from build123d import *

# Parameters (mm, degrees)
CYLINDER002_R     = 18.75
CYLINDER002_DEPTH = 1.4
CYLINDER001_R     = 18.6
CYLINDER001_DEPTH = 2.2
SKETCH_R          = 18.7
PAD_DEPTH         = 24
SKETCH001_R       = 16
PAD001_DEPTH      = 30
SKETCH002_R       = 1
PAD002_DEPTH      = 12
SKETCH003_R       = 13
PAD003_DEPTH      = 16
SKETCH004_R       = 17.5
PAD004_DEPTH      = 11
SKETCH008_R       = 22
SKETCH008_R_2     = 12
PAD008_DEPTH      = 2.5
SKETCH007_R       = 22
SKETCH007_R_2     = 12
PAD007_DEPTH      = 2.5
SKETCH006_R       = 22
SKETCH006_R_2     = 16
PAD006_DEPTH      = 2.5
SKETCH005_R       = 22
SKETCH005_R_2     = 16
PAD005_DEPTH      = 2.5
CYLINDER_R        = 20
CYLINDER_DEPTH    = 93


with BuildPart() as obj1:
    # Cylinder002 → Cylinder002 (new body)
    with BuildSketch(Plane.XY.offset(90)):
        Circle(CYLINDER002_R)
    extrude(amount=CYLINDER002_DEPTH)


with BuildPart() as nut_radial:
    # Cylinder001 → Cylinder001 (new body)
    with BuildSketch(Plane.XY.offset(84)):
        Circle(CYLINDER001_R)
    extrude(amount=CYLINDER001_DEPTH)


with BuildPart() as obj2:
    # Sketch → Pad (new body)
    with BuildSketch(Plane.XY):
        Circle(SKETCH_R)
    extrude(amount=PAD_DEPTH)

    # Sketch001 → Pad001 (new body)
    with BuildSketch(Plane.XY.offset(24)):
        Circle(SKETCH001_R)
    extrude(amount=PAD001_DEPTH)

    # Sketch002 → Pad002 (new body)
    with BuildSketch(Plane.XY.offset(54)):
        with Locations((-9.2, 0)):
            Circle(SKETCH002_R)
    extrude(amount=PAD002_DEPTH)

    # Sketch003 → Pad003 (new body)
    with BuildSketch(Plane.XY.offset(66)):
        Circle(SKETCH003_R)
    extrude(amount=PAD003_DEPTH)

    # Sketch004 → Pad004 (new body)
    with BuildSketch(Plane.XY.offset(82)):
        Circle(SKETCH004_R)
    extrude(amount=PAD004_DEPTH)


with BuildPart() as pad008:
    # Sketch008 → Pad008 (new body)
    with BuildSketch(Plane.XY.offset(56)):
        Circle(SKETCH008_R)
        Circle(SKETCH008_R_2, mode=Mode.SUBTRACT)
    extrude(amount=PAD008_DEPTH)


with BuildPart() as pad007:
    # Sketch007 → Pad007 (new body)
    with BuildSketch(Plane.XY.offset(61)):
        Circle(SKETCH007_R)
        Circle(SKETCH007_R_2, mode=Mode.SUBTRACT)
    extrude(amount=PAD007_DEPTH)


with BuildPart() as pad006:
    # Sketch006 → Pad006 (new body)
    with BuildSketch(Plane.XY.offset(71)):
        Circle(SKETCH006_R)
        Circle(SKETCH006_R_2, mode=Mode.SUBTRACT)
    extrude(amount=PAD006_DEPTH)


with BuildPart() as pad005:
    # Sketch005 → Pad005 (new body)
    with BuildSketch(Plane.XY.offset(66)):
        Circle(SKETCH005_R)
        Circle(SKETCH005_R_2, mode=Mode.SUBTRACT)
    extrude(amount=PAD005_DEPTH)


with BuildPart() as cut012:
    # Cylinder → Cylinder (new body)
    with BuildSketch(Plane.XY):
        Circle(CYLINDER_R)
    extrude(amount=CYLINDER_DEPTH)

    # Cut: cut Pad005
    add(pad005.part, mode=Mode.SUBTRACT)

    # Cut001: cut Pad006
    add(pad006.part, mode=Mode.SUBTRACT)

    # Cut002: cut Pad007
    add(pad007.part, mode=Mode.SUBTRACT)

    # Cut003: cut Pad008
    add(pad008.part, mode=Mode.SUBTRACT)

    # Cut010: cut obj2
    add(obj2.part, mode=Mode.SUBTRACT)

    # Cut011: cut Nut Radial
    add(nut_radial.part, mode=Mode.SUBTRACT)

    # Cut012: cut obj1
    add(obj1.part, mode=Mode.SUBTRACT)


solid = cut012.part
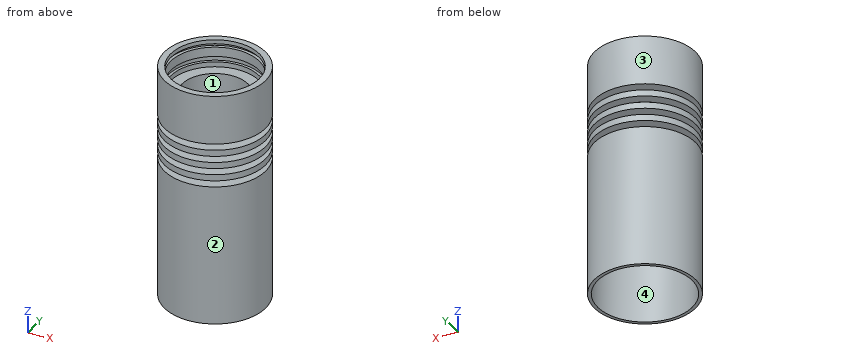
Input: part model. Units: mm. Frame: model coordinates. Face numbers are marked on the shaded views. A direction names the side the tool comes from. Give positions to 0.01 mm unless a question says otherwise; leave off trailing zeros. Order: outer loops, then holes, each group sorted by start corner. A loop starts at its lowest first (then second) coordinate and runs counter-clockwise, first axis right, second up.
Q1. Set-up query: the marked faces 3 and 4. Return all of +Z, -Z, +X, -X, +Y, -Y with unobstructed straight access to the full face (end or side cutting, diameter ignored); none if empty.
Checked values:
face 3: +Z, -Z
face 4: -Z
Q2. Ray query, probe 1 along Z at (x, y) = (14.5, 8); probe 2 along Z at (x, y) = (-3.5, 15.5); probe 3 along Z at (x, y) = (-17.5, 8.5). Return the intervals inside material, ascending.
Checked values:
probe 1: z = 24 to 56, 58.5 to 61, 63.5 to 66, 68.5 to 71, 73.5 to 82
probe 2: z = 54 to 56, 58.5 to 61, 63.5 to 82
probe 3: z = 0 to 56, 58.5 to 61, 63.5 to 66, 68.5 to 71, 73.5 to 93
Q3. Contact query for flat-ended pins moving along their axis: pin 1 Ø6 at (x, z) = (-0.5, 38) entering from -Y; pin 2 Ø12 at (x, y) = (-11, -3) entering from -Z; pin 3 Ø6 at (y, z) = (-3.5, 67.5) entering from +X. Output: stop coordinate, or through.
Checked values:
pin 1: stops at y = -20
pin 2: stops at z = 24
pin 3: stops at x = 19.99
Q4. Section B-B on x = 14.5. State how many separate pieces and enclosed holes the cut face has, and give its area (3 significant figures).
Checked values:
separate pieces: 3
enclosed holes: 0
area: 1,150 mm2
Q5. Draft query along X for the marked faces 1 and 2. Return one class per face: +X half, -X half, draft (parallel to the pull), parting line (faces both ways), or undercut.
Checked values:
face 1: undercut
face 2: parting line
Q6. Section A-A on z = 22. Output: boundary loops of the cut face in (x, y).
Checked values:
outline: circle Ø40 at (0, 0); hole circle Ø37.4 at (0, 0)
Q7. Section D-D on z = 80.5. Output: boundary loops of the cut face in (x, y), and give its area (3 significant figures).
Checked values:
outline: circle Ø40 at (0, 0); hole circle Ø26 at (0, 0)
area: 726 mm2
